```python
from build123d import *

# Parameters (mm, degrees)
SKETCH_1_R          = 2
EXTRUDE_2_DEPTH     = 5
SKETCH_3_W          = 20
SKETCH_3_H          = 8
EXTRUDE_3_DEPTH     = 8
SKETCH_4_R          = 1.9
CUT_EXTRUDE_1_DEPTH = 73.711050963
FILLET_1_R          = 3
FILLET_2_R          = 3
SKETCH_5_W          = 25
SKETCH_5_H          = 10
EXTRUDE_4_DEPTH     = 5
SKETCH_6_W          = 50
SKETCH_6_H          = 4.584747815
EXTRUDE_5_DEPTH     = 2
FILLET_3_R          = 1
FILLET_4_R          = 1
SKETCH_7_R          = 2.45
CUT_EXTRUDE_2_DEPTH = 4
FILLET_5_R          = 1
FILLET_6_R          = 1


with BuildPart() as part:
    # ｽｹｯﾁ1 → ﾎﾞｽ - 押し出し2 (new body)
    with BuildSketch(Plane.XY):
        Polygon((-47, -31.230740592), (-47, -43.230740592), (47, -43.230740592), (47, -31.230740592), (31.5, 2.619259408), (38, 10.369259408), (38, 14.369259408), (-38, 14.369259408), (-38, 10.369259408), (-31.5, 2.619259408), align=None)
        with Locations((-30.5, 8.369259408)):
            Circle(SKETCH_1_R, mode=Mode.SUBTRACT)
        with Locations((30.5, 8.369259408)):
            Circle(SKETCH_1_R, mode=Mode.SUBTRACT)
        with Locations((-37.9, -37.230740592)):
            Circle(SKETCH_1_R, mode=Mode.SUBTRACT)
        with Locations((37.9, -37.230740592)):
            Circle(SKETCH_1_R, mode=Mode.SUBTRACT)
        Polygon((-20, -9.630740592), (-30, -31.230740592), (30, -31.230740592), (20, -9.630740592), align=None, mode=Mode.SUBTRACT)
    extrude(amount=EXTRUDE_2_DEPTH)

    # ｽｹｯﾁ3 → ﾎﾞｽ - 押し出し3 (add)
    with BuildSketch(Plane.XY.offset(5)):
        with Locations((0, -3.230740592)):
            Rectangle(SKETCH_3_W, SKETCH_3_H)
        with Locations((0, -35.230740592)):
            Rectangle(SKETCH_3_W, SKETCH_3_H)
    extrude(amount=EXTRUDE_3_DEPTH)

    # ｽｹｯﾁ4 → ｶｯﾄ - 押し出し1 (cut, through all)
    with BuildSketch(Plane(origin=(10, 0, 0), x_dir=(0, 0, -1), z_dir=(1, 0, 0))):
        with Locations(Location((-9, -3.230740592, 0), (0, 0, 90))):
            Circle(SKETCH_4_R)
        with Locations(Location((-9, -35.230740592, 0), (0, 0, 90))):
            Circle(SKETCH_4_R)
    extrude(amount=-CUT_EXTRUDE_1_DEPTH, mode=Mode.SUBTRACT)

    # ﾌｨﾚｯﾄ1
    fillet_1_edges = [part.edges().sort_by_distance(p)[0] for p in [
        (-30, -31.230740592, 2.5),
        (30, -31.230740592, 2.5),
        (20, -9.630740592, 2.5),
        (-20, -9.630740592, 2.5),
    ]]
    fillet(fillet_1_edges, radius=FILLET_1_R)

    # ﾌｨﾚｯﾄ2
    fillet_2_edges = [part.edges().sort_by_distance(p)[0] for p in [
        (-31.5, 2.619259408, 2.5),
        (31.5, 2.619259408, 2.5),
    ]]
    fillet(fillet_2_edges, radius=FILLET_2_R)

    # ｽｹｯﾁ5 → ﾎﾞｽ - 押し出し4 (add)
    with BuildSketch(Plane.XY.offset(5)):
        with Locations((12.5, -48.230740592)):
            Rectangle(SKETCH_5_W, SKETCH_5_H)
        with Locations((-12.5, -48.230740592)):
            Rectangle(SKETCH_5_W, SKETCH_5_H)
    extrude(amount=-EXTRUDE_4_DEPTH)

    # ｽｹｯﾁ6 → ﾎﾞｽ - 押し出し5 (add)
    with BuildSketch(Plane.XY.offset(5)):
        with Locations((0, -42.938366685)):
            Rectangle(SKETCH_6_W, SKETCH_6_H)
    extrude(amount=EXTRUDE_5_DEPTH)

    # ﾌｨﾚｯﾄ3
    fillet_3_edges = [part.edges().sort_by_distance(p)[0] for p in [
        (-38, 14.369259408, 2.5),
        (38, 14.369259408, 2.5),
    ]]
    fillet(fillet_3_edges, radius=FILLET_3_R)

    # ﾌｨﾚｯﾄ4
    fillet_4_edges = [part.edges().sort_by_distance(p)[0] for p in [
        (47, -43.230740592, 2.5),
        (-47, -43.230740592, 2.5),
    ]]
    fillet(fillet_4_edges, radius=FILLET_4_R)

    # ｽｹｯﾁ7 → ｶｯﾄ - 押し出し2 (cut)
    with BuildSketch(Plane.XY.offset(5)):
        with Locations((-19, -49.230740592)):
            Circle(SKETCH_7_R)
        with Locations((19, -49.230740592)):
            Circle(SKETCH_7_R)
    extrude(amount=-CUT_EXTRUDE_2_DEPTH, mode=Mode.SUBTRACT)

    # ﾌｨﾚｯﾄ5
    fillet_5_edges = [part.edges().sort_by_distance(p)[0] for p in [
        (0, 0.769259408, 5),
        (0, -7.230740592, 5),
    ]]
    fillet(fillet_5_edges, radius=FILLET_5_R)

    # ﾌｨﾚｯﾄ6
    fillet_6_edges = [part.edges().sort_by_distance(p)[0] for p in [
        (0, -39.230740592, 5),
    ]]
    fillet(fillet_6_edges, radius=FILLET_6_R)


solid = part.part
```
The listing builds one solid part. Answer for the finished solid, in the listing's coordinates (mm). A direction names the side the tool comes from. Coordinates: 2 decimals unless noted, no trailing zeros. Write each loop counter-clockwise with the first axis right and the second up, starting at its lowest first coordinate (ties: lowest second). Pieces come first, ordered by that corner, then holes. Notation, with made-up numbers: M -32.75,80 L -7.75,80 A20 cw -7.75,103 Z; hole C 45.5,31.25 d8. An arc over 180 degrees is marked long. Use a Markdown table: item, result. Add a question column.
1. Which of the six approach directions +Z, -Z, +X, -X, +Y, -Y give full straight-line access (tool end or side, diameter ignored) to faces 4 (the cylindrical face through (-19.718, -10.116, 2.535)), 5 (the flat face through (-10, -4, 7)), 6 (the flat face through (0, 0.769, 9)), 7 (the flat face through (-36, -43.231, 2))?
2. For a pull along X with two mould halves and no side action, classify faces 1 (the flat face through (-38, 12, 2)), 2 (the flat face through (-11, -8, 5)), 3 (the cylindrical face through (18.7, -46.8, 3)) as +X half, -X half, draft (parallel to the pull), parting line (faces both ways), or undercut.
3. Section C-C (x = -30.5) is taken. Give the vertices of the cut face in (y, z), plus the area to 3 significant figures.
4. Section D-D (z = 2.25) is taken. Count the separate pieces of the cut face and the enclosed holes in it, plus the area to 3 significant figures.
5. Section B-B (z = 9) is taken. Give the vertices of the cut face in (x, y).
6. Straight lines are drawn through the part: line 1 along Y through (x, z) = (11, 3); line 2 along Y through (x, z) = (30.5, 3.95); line 3 along X through (y, z) = (-36, 4). For each, find the intervals that lie inside material, in ascending order. Write a range as [from, to].
7. Given P1, Ø4, axis at y = -18.5, z = 6, coming from the -X side; P2, Ø1.5, axis at x = 9, z = 11, coming from the -Y side; P3, Ø4.5, axis at x = -19, y = -49.23, coming from the +Z side, each flat-ended and moving along its own axis, determine where each tip first touches the part or whether it passes through.
8. Section A-A (x = 3) is taken. Give the vertices of the cut face in (y, z).
Data:
| question | item | result |
|---|---|---|
| 1 | face 4 | +Z, -Z |
| 1 | face 5 | +Z, -X, +Y |
| 1 | face 6 | +Z, +X, -X, +Y |
| 1 | face 7 | +Z, -Z, -X, -Y |
| 2 | face 1 | -X half |
| 2 | face 2 | draft |
| 2 | face 3 | undercut |
| 3 | outline | M -43.23,0 L 6.37,0 L 6.37,5 L -43.23,5 Z; M 10.37,0 L 14.37,0 L 14.37,5 L 10.37,5 Z |
| 3 | area | 268 mm2 |
| 4 | separate pieces | 1 |
| 4 | enclosed holes | 7 |
| 4 | area | 3,970 mm2 |
| 5 | outline | M -10,-39.23 L 10,-39.23 L 10,-37.13 L -10,-37.13 Z; M -10,-33.33 L 10,-33.33 L 10,-31.23 L -10,-31.23 Z; M -10,-7.23 L 10,-7.23 L 10,-5.13 L -10,-5.13 Z; M -10,-1.33 L 10,-1.33 L 10,0.77 L -10,0.77 Z |
| 6 | line 1 | y = [-53.23, -31.23], [-9.63, 14.37] |
| 6 | line 2 | y = [-43.23, 6.37], [10.37, 14.37] |
| 6 | line 3 | x = [-47, -39.48], [-36.32, 36.32], [39.48, 47] |
| 7 | P1 | stops at x = -41.96 |
| 7 | P2 | stops at y = -39.23 |
| 7 | P3 | stops at z = 1 |
| 8 | outline | M -53.23,0 L -31.23,0 L -31.23,13 L -39.23,13 L -39.23,6 A1 cw -40.23,5 L -40.65,5 L -40.65,7 L -45.23,7 L -45.23,5 L -53.23,5 Z; M -9.63,0 L 14.37,0 L 14.37,5 L 1.77,5 A1 cw 0.77,6 L 0.77,13 L -7.23,13 L -7.23,6 A1 cw -8.23,5 L -9.63,5 Z; hole C -35.23,9 d3.8; hole C -3.23,9 d3.8 |
